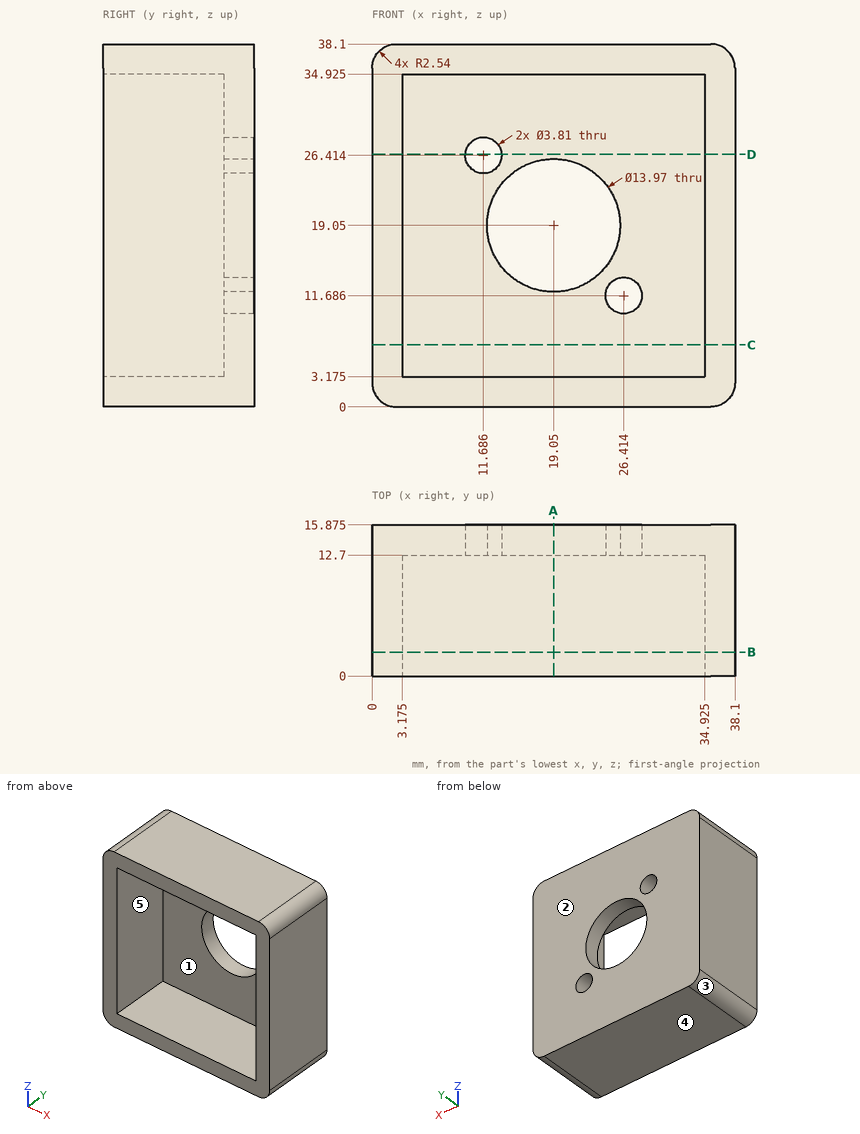
Answer from the drawing. Dimensions are ordinates in mm from the lowest x, y and z of the part. A direction names the side the tool comes from. Round coordinates to 2 decimals unless told otherwise and drop trailing zeros. Loops run counter-clockwise (first coordinate to the right, second up) from the corner with the lowest first, then second, coordinate; pieces in that order, holes last. Notation, with made-up numbers: (16.5, 22) - (75.5, 22) arc R15 cw to (75.5, 41) - close; hole circle Ø5 at (16, 54.25). An arc over 180 degrees is marked (long way). Return JSON: item names as keys, results as strings. Group by question number.
1. The part is cut by section B-B on y = 2.5. Determine the outline of the cut face in (x, z) (3 decimals), then the cut area to 3 significant figures.
2. The part is cut by section C-C on z = 6.5. Determine the outline of the cut face in (x, y) (3 decimals).
3. Each of these flat-tipped pins is pushed along its axis until it touches: P1, Ø5, axis at x = 4, z = 10.5, coming from the -Y side; P2, Ø16, axis at x = 14.5, z = 14, coming from the -Y side. Where does it stop, or does it pass through?
4. The part is cut by section A-A on x = 19.05. Determine the outline of the cut face in (y, z) (3 decimals), then the cut area to 3 significant figures.
5. The part is cut by section D-D on z = 26.5. Determine the outline of the cut face in (x, y) (1 decimal).
6. Consider probe 1 along X at (y, z) = (14, 19.05) (3 decimals); probe 2 along Z at (x, y) = (31, 2.5) (3 decimals). Determine where each line is inside the solid, lowest interval first.
7. Which of the six approach directions +Z, -Z, +X, -X, +Y, -Y give full straight-line access (tool end or side, diameter ignored) to the marked faces 4 and 5?
8. The mould has two halves that part along X. Classify the marked faces 1, 2 and 3: pulls with the +X half, pulls with the -X half, needs draft (parallel to the pull), parting line crosses it, or undercut.
Resolved:
{
 "1": {"outline": "(0, 2.54) arc R2.54 ccw to (2.54, 0) - (35.56, 0) arc R2.54 ccw to (38.1, 2.54) - (38.1, 35.56) arc R2.54 ccw to (35.56, 38.1) - (2.54, 38.1) arc R2.54 ccw to (0, 35.56) - close; hole (3.175, 3.175) - (34.925, 3.175) - (34.925, 34.925) - (3.175, 34.925) - close", "area": "438 mm²"},
 "2": {"outline": "(0, 0) - (3.175, 0) - (3.175, 12.7) - (34.925, 12.7) - (34.925, 0) - (38.1, 0) - (38.1, 15.875) - (0, 15.875) - close"},
 "3": {"P1": "stops at y = 0", "P2": "stops at y = 12.7"},
 "4": {"outline": "(0, 0) - (15.875, 0) - (15.875, 12.065) - (12.7, 12.065) - (12.7, 3.175) - (0, 3.175) - close; (0, 34.925) - (12.7, 34.925) - (12.7, 26.035) - (15.875, 26.035) - (15.875, 38.1) - (0, 38.1) - close", "area": "157 mm²"},
 "5": {"outline": "(0, 0) - (3.2, 0) - (3.2, 12.7) - (9.8, 12.7) - (9.8, 15.9) - (0, 15.9) - close; (13.6, 12.7) - (34.9, 12.7) - (34.9, 0) - (38.1, 0) - (38.1, 15.9) - (13.6, 15.9) - close"},
 "6": {"probe 1": "x = 0 to 12.065, 26.035 to 38.1", "probe 2": "z = 0 to 3.175, 34.925 to 38.1"},
 "7": {"face 4": "-Z, +X, -X, +Y, -Y", "face 5": "-Y"},
 "8": {"face 1": "undercut", "face 2": "needs draft", "face 3": "pulls with the -X half"}
}
